from build123d import *

# Parameters (mm, degrees)
SKETCH1_W           = 200
SKETCH1_H           = 150
BOSS_EXTRUDE1_DEPTH = 20
BOSS_EXTRUDE2_DEPTH = 50
CUT_EXTRUDE1_DEPTH  = 25
SKETCH6_R           = 20
CUT_EXTRUDE2_DEPTH  = 126


with BuildPart() as part:
    # Sketch1 → Boss-Extrude1 (new body)
    with BuildSketch(Plane(origin=(0, 0, 0), x_dir=(1, 0, 0), z_dir=(0, 1, 0))):
        Rectangle(SKETCH1_W, SKETCH1_H)
    extrude(amount=BOSS_EXTRUDE1_DEPTH)

    # Sketch3 → Boss-Extrude2 (add, symmetric)
    with BuildSketch(Plane.XY):
        with BuildLine():
            Line((-37.997361363, 132.498021022), (-75, 20))
            Line((-75, 20), (75, 20))
            Line((75, 20), (37.997361363, 132.498021022))
            ThreePointArc((37.997361363, 132.498021022), (0, 160), (-37.997361363, 132.498021022))
        make_face()
    extrude(amount=BOSS_EXTRUDE2_DEPTH, both=True)

    # Sketch5 → Cut-Extrude1 (cut, symmetric)
    with BuildSketch(Plane.XY):
        with BuildLine():
            Line((-37.997361363, 132.498021022), (-75, 20))
            Line((-75, 20), (75, 20))
            Line((75, 20), (37.997361363, 132.498021022))
            ThreePointArc((37.997361363, 132.498021022), (0, 160), (-37.997361363, 132.498021022))
        make_face()
    extrude(amount=CUT_EXTRUDE1_DEPTH, both=True, mode=Mode.SUBTRACT)

    # Sketch6 → Cut-Extrude2 (cut, through all)
    with BuildSketch(Plane.XY.offset(50)):
        with Locations((0, 120)):
            Circle(SKETCH6_R)
    extrude(amount=-CUT_EXTRUDE2_DEPTH, mode=Mode.SUBTRACT)


solid = part.part
Can you work these out from the model? Positions are in its coordinate system, mm. A direction names the side the tool comes from. Coordinates: 2 decimals unless noted, no trailing zeros. Write each loop counter-clockwise with the first axis right and the second up, starting at its lowest first coordinate (ties: lowest second). Pieces come first, ordered by that corner, then holes. Notation, with made-up numbers: (-14, -40) - (3, -40) arc R30 cw to (3, -5) - close; hole circle Ø8 at (-27.75, 51). An arc over 180 degrees is marked (long way). Return JSON: item names as keys, results as strings. Group by question number.
Item 1: We'd pull the mould along Z, two halves only. Please class faces 1 (the face through (-1, 10, 75)), 2 (the face through (-1, 75, 25)), 3 (the face through (-4.336, 100.476, -37.325)): pulls with the +Z half, pulls with the -Z half, needs draft (parallel to the pull), parting line crosses it, or undercut.
Item 2: If we section it at B-B (z = -36.5): Write out the boundary of the cut face in (x, y), then the cut area to 3 significant figures.
Item 3: If we section it at D-D (x = -44): Write out the boundary of the cut face in (y, z), then the cut area to 3 significant figures.
Item 4: If we section it at C-C (y = 104): Write out the boundary of the cut face in (x, z).
Item 5: I'm going to push flat-ended pins straight in: pin 1 Ø1.5 at (x, z) = (8.5, -46) entering from +Y; pin 2 Ø2 at (x, y) = (-27, 93.5) entering from +Z; pin 3 Ø5 at (x, z) = (2.5, 10.5) entering from +Y. Where does each tip first touch, or does it pass through?
Item 6: Which directions (+Z, -Z, +X, -X, +Y, -Y) give clear straight access to the entire face, cutting with the end or side of a thin tool? Please do faces 4 (the face through (-1, 75, -25)), 5 (the face through (56.76, 75.46, -37.33)), 6 (the face through (-1, 75, -50)), 7 (the face through (-1, 75, 50)), 8 (the face through (0.702, 159.994, 37.675)).
Item 7: If we section it at A-A (x = 0): Write out the boundary of the cut face in (y, z).
Item 8: Please list where these lines run through material, in increasing order: probe 1 along Z at (x, y) = (-22.5, 43); probe 2 along Y at (x, z) = (-26, -17); probe 3 along X at (y, z) = (60, -26).
Return value:
{
 "1": {"face 1": "pulls with the +Z half", "face 2": "undercut", "face 3": "needs draft"},
 "2": {"outline": "(-100, 0) - (100, 0) - (100, 20) - (75, 20) - (38, 132.5) arc R40 ccw to (-38, 132.5) - (-75, 20) - (-100, 20) - close; hole circle Ø40 at (0, 120)", "area": "17,000 mm^2"},
 "3": {"outline": "(0, -75) - (20, -75) - (20, -50) - (114.25, -50) - (114.25, -25) - (20, -25) - (20, 25) - (114.25, 25) - (114.25, 50) - (20, 50) - (20, 75) - (0, 75) - close", "area": "7,710 mm^2"},
 "4": {"outline": "(-47.37, -50) - (-12, -50) - (-12, -25) - (-47.37, -25) - close; (-47.37, 25) - (-12, 25) - (-12, 50) - (-47.37, 50) - close; (12, -50) - (47.37, -50) - (47.37, -25) - (12, -25) - close; (12, 25) - (47.37, 25) - (47.37, 50) - (12, 50) - close"},
 "5": {"pin 1": "stops at y = 159.24", "pin 2": "stops at z = 50", "pin 3": "stops at y = 20"},
 "6": {"face 4": "+X, -X, +Y", "face 5": "+Z, -Z, +X, +Y", "face 6": "-Z, +X, -X, +Y", "face 7": "+Z, +X, -X, +Y", "face 8": "+Z, -Z, +Y"},
 "7": {"outline": "(0, -75) - (20, -75) - (20, -50) - (100, -50) - (100, -25) - (20, -25) - (20, 25) - (100, 25) - (100, 50) - (20, 50) - (20, 75) - (0, 75) - close; (140, -50) - (160, -50) - (160, -25) - (140, -25) - close; (140, 25) - (160, 25) - (160, 50) - (140, 50) - close"},
 "8": {"probe 1": "z = -50 to -25, 25 to 50", "probe 2": "y = 0 to 20", "probe 3": "x = -61.84 to 61.84"}
}
